Geometry check sheet. Reference: the model listing, model coordinates, mm. A direction names the side the tool comes from. Give positions to 0.01 mm unless a question says otherwise; leave off trailing zeros. Order: outer loops, then holes, each group sorted by start corner. A loop starts at its lowest first (then second) coordinate and runs counter-clockwise, first axis right, second up. Notation, with made-up numbers: M -36,30 L -23,30 A26 ccw -23,46 Z; hole C 82.25,68.25 d7. An arc over 180 degrees is marked long. Answer as CSV lines item,"result".
Autodesk Inventor part; units mm, degrees
ref_plane "to_bolt_XY" through (1.9, 0, 0) normal (1, 0, 0) x (0, 0, -1)
ref_plane "to_bolt_YZ" through (1.9, 0, 0) normal (0, 0, -1) x (0, 1, 0)
ref_plane "to_bolt_ZX" through (1.9, 0, 0) normal (0, 1, 0) x (1, 0, 0)
sketch "Sketch_1" plane through (0, 0, 0) normal (0, 0, 1) x (1, 0, 0)
  line L0 (1.9, 0) -> (-1.1, 0)
  line L1 (-1.1, 0) -> (-1.1, 2.75)
  line L2 (-1.1, 2.75) -> (-1.9, 2.75)
  line L3 (-1.9, 2.75) -> (-1.9, 3.3)
  arc A0 (-1.7, 3.5) -> (-1.9, 3.3) centre (-1.7, 3.3) ccw
  line L4 (-1.7, 3.5) -> (-1.1, 3.5)
  line L5 (-1.1, 3.5) -> (-0.9526, 4.05)
  line L6 (-0.9526, 4.05) -> (1.7526, 4.05)
  line L7 (1.7526, 4.05) -> (1.9, 3.5)
  line L8 (1.9, 3.5) -> (1.9, 0)
  line L9 (1.9, 0) -> (-1.1, 0)
revolve "Revolution1" add sketch "Sketch_1" angle 360 about axis through (1.9, 0, 0) along (1, 0, 0)
sketch "Sketch_2" plane through (0, 0, 0) normal (1, 0, 0) x (0, 1, 0)
  line L0 (7, 7) -> (-7, 7)
  line L1 (-7, 7) -> (-7, -7)
  line L2 (-7, -7) -> (7, -7)
  line L3 (7, -7) -> (7, 7)
  line L4 (-2.0207, 3.5) -> (-4.0415, 0)
  line L5 (-4.0415, 0) -> (-2.0207, -3.5)
  line L6 (-2.0207, -3.5) -> (2.0207, -3.5)
  line L7 (2.0207, -3.5) -> (4.0415, 0)
  line L8 (4.0415, 0) -> (2.0207, 3.5)
  line L9 (2.0207, 3.5) -> (-2.0207, 3.5)
extrude "Extrusion1" cut sketch "Sketch_2" along normal mid plane 3.8
sketch "Sketch_3" plane through (0, 0, 0) normal (0, 0, 1) x (1, 0, 0)
  line L0 (1.9, 0) -> (-1.1, 0)
  line L1 (-1.1, 0) -> (-1.1, 2)
  line L2 (-1.1, 2) -> (-0.721, 1.621)
  line L3 (-0.721, 1.621) -> (1.521, 1.621)
  line L4 (1.521, 1.621) -> (1.9, 2)
  line L5 (1.9, 2) -> (1.9, 0)
  line L6 (1.9, 0) -> (-1.1, 0)
revolve "Revolution2" cut sketch "Sketch_3" angle 360 about axis through (1.9, 0, 0) along (1, 0, 0)
thread "Thread1"
sketch "Sketch_7" plane through (-1.1, 0, 0) normal (1, 0, 0) x (0, 0, -1)
  line L0 (-1.375, 2.3816) -> (-0.8, 1.3856)
  arc A0 (0.8, 1.3856) -> (-0.8, 1.3856) centre (0, 0) ccw
  line L1 (0.8, 1.3856) -> (1.375, 2.3816)
  arc A1 (1.375, 2.3816) -> (-1.375, 2.3816) centre (0, 0) ccw
extrude "Extrusion2" add sketch "Sketch_7" against normal blind 0.4
sketch "Sketch_9" plane through (-1.1, 0, 0) normal (1, 0, 0) x (0, 0, -1)
  arc A0 (-2.75, 0) -> (-1.375, -2.3816) centre (0, 0) ccw
  line L0 (-1.375, -2.3816) -> (-0.8, -1.3856)
  arc A1 (-1.6, 0) -> (-0.8, -1.3856) centre (0, 0) ccw
  line L1 (-1.6, 0) -> (-2.75, 0)
extrude "Extrusion3" add sketch "Sketch_9" against normal blind 0.4
sketch "Sketch_8" plane through (-1.1, 0, 0) normal (1, 0, 0) x (0, 0, -1)
  line L0 (0.8, -1.3856) -> (1.375, -2.3816)
  arc A0 (1.375, -2.3816) -> (2.75, 0) centre (0, 0) ccw
  line L1 (2.75, 0) -> (1.6, 0)
  arc A1 (0.8, -1.3856) -> (1.6, 0) centre (0, 0) ccw
extrude "Extrusion4" add sketch "Sketch_8" against normal blind 0.4
ref_plane "to_bolt_XY" through (1.9, 0, 0) normal (1, 0, 0) x (0, 0, -1)
ref_plane "to_bolt_YZ" through (1.9, 0, 0) normal (0, 0, -1) x (0, 1, 0)
ref_plane "to_bolt_ZX" through (1.9, 0, 0) normal (0, 1, 0) x (1, 0, 0)
properties part number "UNUTZ4"
(1) Draft check along Z on faces 1 (the face through (-1.06, 3.65, -0.08)), 2 (the face through (0.4, 3, -1.8)), 3 (the face through (0.379, 3.045, 1.726)), 4 (the face through (-1.594, -2.747, -0.121)). Enter one of: +Z half, -Z half, draft (parallel to the pull), parting line (faces both ways), or undercut.
The answers:
face 1,"parting line"
face 2,"-Z half"
face 3,"+Z half"
face 4,"undercut"
(2) Material ranges on line 1 (Z direction, x = 0.5, y = 0); line 2 (Y direction, x = 0.6, z = -1.75); line 3 (Y direction, x = -1.3, z = 0.75), recorded low to high.
The answers:
line 1,"z = -3.5 to -1.62, 1.62 to 3.5"
line 2,"y = -3.03 to 3.03"
line 3,"y = -3.42 to -2.65, 1.41 to 3.42"
(3) Gauge pin test, flat ends, axial feed: P1, Ø4, axis at y = 0, z = 0, coming from the -X side; P2, Ø0.9, axis at y = 1, z = 2, coming from the -X side. Record the tip position at first contact, or that the pin passes through.
The answers:
P1,"stops at x = -1.5"
P2,"stops at x = -1.1"
(4) Section check A-A on x = -0.4. Enter the section's corners in (y, z), then the cut area to 3 significant figures.
The answers:
outline,"M -4.04,0 L -2.02,-3.5 L 2.02,-3.5 L 4.04,0 L 2.02,3.5 L -2.02,3.5 Z; hole C 0,0 d3.24"
area,"34.2 mm2"
(5) Tool access check on faces 5 (the face through (1.85, -1.85, 3.19)), 6 (the face through (-1.5, -1, -2)), 7 (the face through (0.416, 0.748, -1.438)). Record the directions out of +Z, -Z, +X, -X, +Y, -Y that give a thin tool (end or side, any length) a straight path to the whole face; none if there is none.
The answers:
face 5,"+Z, +X, -Y"
face 6,"-X"
face 7,"+X"
